Autodesk Inventor part; units mm, degrees
ref_plane "YZ Plane" through (0, 0, 0) normal (1, 0, 0) x (0, 1, 0)
ref_plane "XZ Plane" through (0, 0, 0) normal (0, 1, 0) x (-1, 0, 0)
ref_plane "XY Plane" through (0, 0, 0) normal (0, 0, 1) x (1, 0, 0)
sketch "Sketch1" plane through (0, 0, 0) normal (0, 0, 1) x (1, 0, 0)
  line L0 (-5.5, 3.5) -> (5.5, 3.5)
  line L1 (5.5, 3.5) -> (5.5, -3.5)
  line L2 (5.5, -3.5) -> (-5.5, -3.5)
  line L3 (-5.5, -3.5) -> (-5.5, 3.5)
  line L4 (-5.5, 3.5) -> (5.5, -3.5) construction
  line L5 (5.5, 3.5) -> (-5.5, -3.5) construction
  point P0 (0, 0)
  dimension "d0" = 11
  dimension "d1" = 7
extrude "Extrusion1" add sketch "Sketch1" along normal blind 20
sketch "Sketch2" plane through (0, 0, 20) normal (0, 0, 1) x (1, 0, 0)
  circle A0 centre (0, 0) radius 3.25
  dimension "d4" = 6.5
extrude "Extrusion2" add sketch "Sketch2" along normal blind 4.8
fillet "Fillet1" radius 2 5 edges at (5.5, 3.5, 10) (5.5, -3.5, 10) (-5.5, 3.5, 10) (-5.5, -3.5, 10) (-3.25, 0, 20)
properties part number "Cable_Usb_C"
CAD build for the part. Positions are in the model's coordinates, mm. A direction names the side the tool comes from. Round coordinates to 2 decimals unless told otherwise and drop trailing zeros. Order: outer loops, then holes, each group sorted by start corner. A loop starts at its lowest first (then second) coordinate and runs counter-clockwise, first axis right, second up. Notation, with made-up numbers: (85.5, 18.25) - (139.5, 18.25) arc R22 ccw to (139.5, 44.25) - close; hole circle Ø7 at (52, 37.5). An arc over 180 degrees is marked (long way). Use CSV: the item, a comma, the result in double quotes. Start each with the question number.
1) Wall check: L1, parallel to Z at x = 5, y = -2; L2, parallel to Z at x = -3.75, y = 2.5; L3, parallel to X at y = 3.25, z = 8.5. Give the ranges that are in metal, low to high. Write a range as [from, to].
2) Saw through at C-C (z = 23.25). List the corners of the cut face in (x, y).
3) Saw through at A-A (y = 0). List the corners of the cut face in (x, z), and give its area (3 significant figures).
4) Pin check, flat tips, straight feed: pin 1 Ø1 at (x, z) = (3.5, 21) entering from -Y; pin 2 Ø1.7 at (x, y) = (4.5, 1) entering from +Z; pin 3 Ø0.8 at (x, y) = (-5, -1) entering from +Z. Stop position of each tip, or through.
5) Tool access for faces 1 (the cylindrical face through (-2.579, 1.978, 23.38)), 2 (the flat face through (0, -3.5, 10)): list every direction of +Z, -Z, +X, -X, +Y, -Y with a clear straight run to the whole face (end or side of a thin tool).
6) Saw through at B-B (z = 5.5). List the corners of the cut face in (x, y), and give its area (3 significant figures).
Values follow:
1,L1,"z = [0, 20]"
1,L2,"z = [0, 20.14]"
1,L3,"x = [-4.47, 4.47]"
2,outline,"circle Ø6.5 at (0, 0)"
3,outline,"(-5.5, 0) - (5.5, 0) - (5.5, 20) - (5.25, 20) arc R2 cw to (3.25, 22) - (3.25, 24.8) - (-3.25, 24.8) - (-3.25, 22) arc R2 cw to (-5.25, 20) - (-5.5, 20) - close"
3,area,"253 mm2"
4,pin 1,"stops at y = -2.09"
4,pin 2,"stops at z = 20.67"
4,pin 3,"stops at z = 20.08"
5,face 1,"+Z"
5,face 2,"+Z, -Z, +X, -X, -Y"
6,outline,"(-5.5, -1.5) arc R2 ccw to (-3.5, -3.5) - (3.5, -3.5) arc R2 ccw to (5.5, -1.5) - (5.5, 1.5) arc R2 ccw to (3.5, 3.5) - (-3.5, 3.5) arc R2 ccw to (-5.5, 1.5) - close"
6,area,"73.6 mm2"
